Geometry check sheet. Reference: the model listing, model coordinates, mm. A direction names the side the tool comes from. Round coordinates to 2 decimals unless told otherwise and drop trailing zeros. Loops run counter-clockwise (first coordinate to the right, second up) from the corner with the lowest first, then second, coordinate; pieces in that order, holes last. Notation, with made-up numbers: M 3.5,84.5 L 60.5,84.5 A28 cw 60.5,114.5 Z; hole C 15.25,0.5 d1. An arc over 180 degrees is marked long. Answer in a Markdown table with one row per item. Add a question column.
```python
from build123d import *

# Parameters (mm, degrees)
SKETCH1_W               = 6
SKETCH1_H               = 4
SKETCH1_W_2             = 9
SKETCH1_W_3             = 10
SKETCH1_H_2             = 6
SKETCH2_R               = 3
CUT_EXTRUDE3_DEPTH      = 10
CUT_EXTRUDE3_DEPTH_BACK = 10


with BuildPart() as part:
    # Sketch1 → Revolve1 (revolve)
    with BuildSketch(Plane.XY):
        Polygon((0, 6), (0, 0), (7, 0), (7, 4), (7, 6), align=None)
        with Locations((10, 2)):
            Rectangle(SKETCH1_W, SKETCH1_H)
        with Locations((17.5, 2)):
            Rectangle(SKETCH1_W_2, SKETCH1_H)
        Polygon((22, 4), (22, 0), (104, 0), (104, 6), (104, 8), (22, 8), align=None)
        with Locations((109, 3)):
            Rectangle(SKETCH1_W_3, SKETCH1_H_2)
        Polygon((114, 6), (114, 0), (138, 0), (138, 9), (114, 9), align=None)
    revolve(axis=Axis((0, 0, 0), (1, 0, 0)))

    # Sketch2 → Cut-Extrude3 (cut, two sides)
    with BuildSketch(Plane(origin=(0, 0, 0), x_dir=(1, 0, 0), z_dir=(0, 1, 0))) as cut_extrude3_sk:
        with Locations((126, 0)):
            Circle(SKETCH2_R)
    extrude(amount=CUT_EXTRUDE3_DEPTH, mode=Mode.SUBTRACT)
    extrude(cut_extrude3_sk.sketch, amount=-CUT_EXTRUDE3_DEPTH_BACK, mode=Mode.SUBTRACT)


solid = part.part
```
1) Thickness scan on L1, parallel to X at y = 5, z = 0; L2, parallel to X at y = -6, z = -1.75; L3, parallel to X at y = -8, z = -3.25. Record the ranges inside material, lowest first. Write a range as [from, to].
2) Set-up check for faces 1 (the flat face through (0, 0, 0)), 2 (the flat face through (114, 2, -6)), 3 (the cylindrical face through (3, -6, 0)): record each of +Z, -Z, +X, -X, +Y, -Y from which the full face is reachable in a straight line by a thin tool's end or side.
3) Go/stop test with flat-tipped pins: pin 1 (5 mm diameter, centred on x = 33, y = -6, fed in from +Z); pin 2 (1 mm diameter, centred on x = 26.5, z = 4, fed in from +Y); pin 3 (5 mm diameter, centred on x = 126, z = 0, fed in from -Y). Record where each tip stops, or that it passes through.
4) Cross-section at A-A, the plane z = 0. Record the boundary of the cut face in (x, y), plus the area to 3 significant figures.
5) Cross-section at C-C, the plane x = 126. Record the boundary of the cut face in (y, z).
6) Cross-section at B-B, the plane y = 2.75. Record the boundary of the cut face in (x, z).
7) Draft check along X on faces 4 (the cylindrical face through (109, -6, 0)), 5 (the flat face through (7, 1.42, -3.92)), 6 (the flat face through (138, 0, 0)), 7 (the cylindrical face through (62.43, -1.73, -7.81)). Enter one of: +X half, -X half, draft (parallel to the pull), parting line (faces both ways), or undercut.
8) Cross-section at D-D, the plane x = 72. Record the boundary of the cut face in (y, z).
Worked answers:
| question | item | result |
|---|---|---|
| 1 | L1 | x = [0, 7], [22, 123], [129, 138] |
| 1 | L2 | x = [22, 104], [114, 123.56], [128.44, 138] |
| 1 | L3 | x = [114, 138] |
| 2 | face 1 | +Z, -Z, -X, +Y, -Y |
| 2 | face 2 | none |
| 2 | face 3 | -X |
| 3 | pin 1 | stops at z = 7.19 |
| 3 | pin 2 | stops at y = 7.19 |
| 3 | pin 3 | passes through |
| 4 | outline | M 0,-6 L 7,-6 L 7,-4 L 22,-4 L 22,-8 L 104,-8 L 104,-6 L 114,-6 L 114,-9 L 123,-9 L 123,9 L 114,9 L 114,6 L 104,6 L 104,8 L 22,8 L 22,4 L 7,4 L 7,6 L 0,6 Z; M 129,-9 L 138,-9 L 138,9 L 129,9 Z |
| 4 | area | 1,960 mm2 |
| 5 | outline | M -8.49,-3 A9 ccw 8.49,-3 Z; M -8.49,3 L 8.49,3 A9 ccw Z |
| 6 | outline | M 0,-5.33 L 7,-5.33 L 7,-2.9 L 22,-2.9 L 22,-7.51 L 104,-7.51 L 104,-5.33 L 114,-5.33 L 114,-8.57 L 138,-8.57 L 138,8.57 L 114,8.57 L 114,5.33 L 104,5.33 L 104,7.51 L 22,7.51 L 22,2.9 L 7,2.9 L 7,5.33 L 0,5.33 Z; hole C 126,0 d6 |
| 7 | face 4 | undercut |
| 7 | face 5 | undercut |
| 7 | face 6 | +X half |
| 7 | face 7 | draft |
| 8 | outline | C 0,0 d16 |
